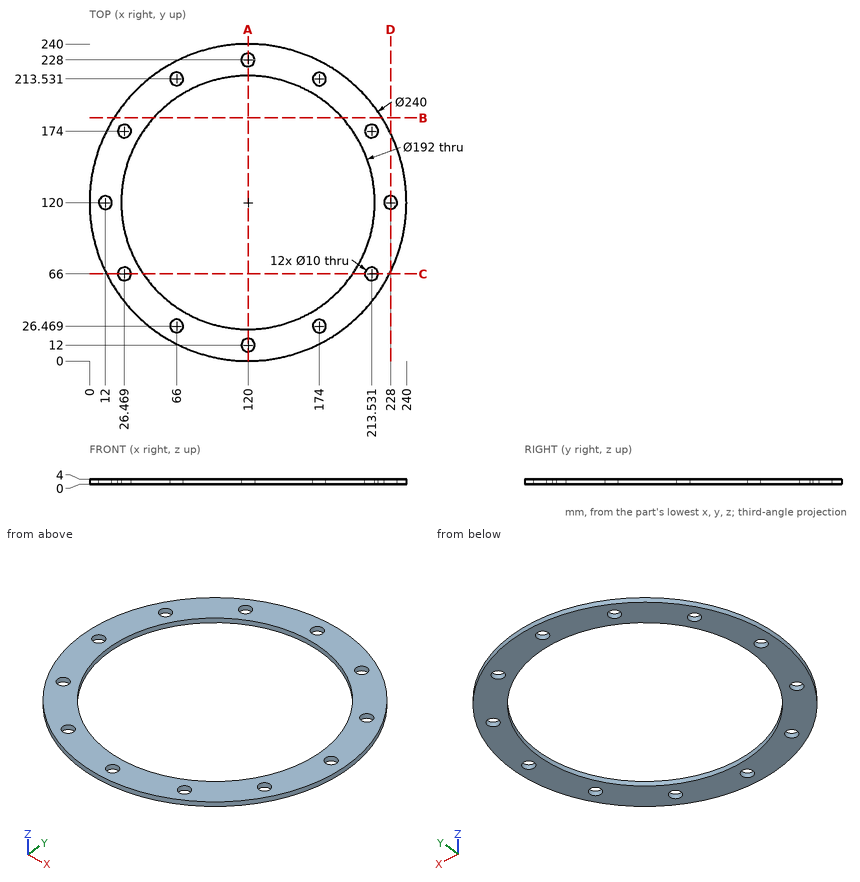
Source: three-view drawing plus pictorial views. Frame: mm from the lowest corner of the part. Coordinates: 2 decimals unless noted, no trailing zeros. Write each loop counter-clockwise with the first axis right and the second up, starting at its lowest first coordinate (ties: lowest second). Pieces come first, ordered by that corner, then holes. Notation, with made-up numbers: (39.5, -40) - (70.5, -40) arc R36 cw to (70.5, -4) - close; hole circle Ø8 at (42, 55). An arc over 180 degrees is marked (long way). Answer as a JSON object with one key per item and string values.
Q1. Section query A-A, the plane x = 120. Output: boundary loops of the cut face in (y, z).
Ans:
{"outline": "(0, 0) - (7, 0) - (7, 4) - (0, 4) - close; (17, 0) - (24, 0) - (24, 4) - (17, 4) - close; (216, 0) - (223, 0) - (223, 4) - (216, 4) - close; (233, 0) - (240, 0) - (240, 4) - (233, 4) - close"}
Q2. First-contact query: pin 1 Ø2 at (x, z) = (84, 2) entering from -Y; pin 2 Ø12 at (x, y) = (35.5, 111.5) entering from +Z. Flat tips, straight axial feed; report the tip coordinate or a pass-through.
Ans:
{"pin 1": "stops at y = 5.22", "pin 2": "passes through"}
Q3. Section query C-C, the plane y = 66. Output: boundary loops of the cut face in (x, z).
Ans:
{"outline": "(12.84, 0) - (21.47, 0) - (21.47, 4) - (12.84, 4) - close; (31.47, 0) - (40.63, 0) - (40.63, 4) - (31.47, 4) - close; (199.37, 0) - (208.53, 0) - (208.53, 4) - (199.37, 4) - close; (218.53, 0) - (227.16, 0) - (227.16, 4) - (218.53, 4) - close"}
Q4. Section query D-D, the plane x = 228. Output: boundary loops of the cut face in (y, z).
Ans:
{"outline": "(67.69, 0) - (115, 0) - (115, 4) - (67.69, 4) - close; (125, 0) - (172.31, 0) - (172.31, 4) - (125, 4) - close"}
Q5. Section query B-B, the plane y = 184. Output: boundary loops of the cut face in (x, z).
Ans:
{"outline": "(18.49, 0) - (48.45, 0) - (48.45, 4) - (18.49, 4) - close; (191.55, 0) - (221.51, 0) - (221.51, 4) - (191.55, 4) - close"}
Q6. Material intervals for line 1 (X direction, y = 68, z = 0.7); line 2 (Y direction, x = 168.5, z = 2.35); line 3 (X direction, y = 138.5, z = 3.7) (1 decimal), sorted ascending. Write a range as [from, to].
Ans:
{"line 1": "x = [11.85, 21.89], [31.05, 39.3], [200.7, 208.95], [218.11, 228.15]", "line 2": "y = [10.24, 37.15], [202.85, 229.76]", "line 3": "x = [1.4, 25.8], [214.2, 238.6]"}
